The listing builds one solid part. Answer for the finished solid, in the listing's coordinates (mm). Face numbers are marked on the shaded views. Coordinates: 2 decimals unless noted, no trailing zeros. Write each loop counter-clockwise with the first axis right and the second up, starting at its lowest first coordinate (ties: lowest second). Pieces come first, ordered by that corner, then holes. Notation, with made-up numbers: M 53,76.25 L 90,76.25 A12 cw 90,99.25 Z; hole C 32.25,75.25 d3. An arc over 180 degrees is marked long. Answer as CSV lines item,"result".
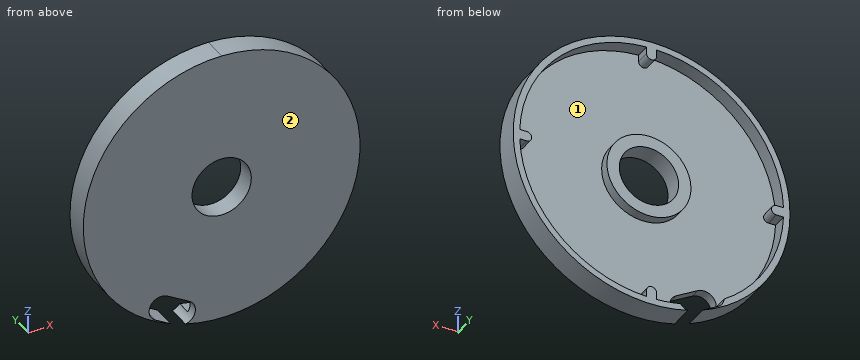
```python
from build123d import *

# Parameters (mm, degrees)
SKETCH_1_R               = 28
EXTRUDE_1_DEPTH          = 2
SKETCH_2_R               = 28
SKETCH_2_R_2             = 26.7
EXTRUDE_3_DEPTH          = 3
EXTRUDE_4_DEPTH          = 3
PATTERN_CIRCULAR_1_COUNT = 4
CUT_EXTRUDE_1_DEPTH      = 5
SKETCH_5_R               = 8.5
SKETCH_5_R_2             = 6
EXTRUDE_5_DEPTH          = 2
SKETCH_6_R               = 6
CUT_EXTRUDE_2_DEPTH      = 2.5


with BuildPart() as part:
    # 草图1 → 凸台-拉伸1 (new body)
    with BuildSketch(Plane(origin=(0, 0, 0), x_dir=(1, 0, 0), z_dir=(0, 1, 0))):
        with Locations(Location((0, 0, 0), (0, 0, 270))):
            Circle(SKETCH_1_R)
    extrude(amount=EXTRUDE_1_DEPTH)

    # 草图2 → 凸台-拉伸3 (add)
    with BuildSketch(Plane(origin=(0, 2, 0), x_dir=(1, 0, 0), z_dir=(0, 1, 0))):
        with Locations(Location((0, 0, 0), (0, 0, 270))):
            Circle(SKETCH_2_R)
        with Locations(Location((0, 0, 0), (0, 0, 270))):
            Circle(SKETCH_2_R_2, mode=Mode.SUBTRACT)
    extrude(amount=EXTRUDE_3_DEPTH)

    # 草图3 → 凸台-拉伸4 (add)
    with BuildSketch(Plane(origin=(0, 2, 0), x_dir=(1, 0, 0), z_dir=(0, 1, 0))):
        with BuildLine():
            Line((1, 26.681266836), (1, 25.262759823))
            ThreePointArc((1, 25.262759823), (0, 24.262759823), (-1, 25.262759823))
            Line((-1, 25.262759823), (-1, 26.681266836))
            ThreePointArc((-1, 26.681266836), (0, 26.7), (1, 26.681266836))
        make_face()
    extrude_4 = extrude(amount=EXTRUDE_4_DEPTH)

    # 阵列(圆周)1: 凸台-拉伸4 ×4 about axis
    pattern_circular_1_axis = Axis((0, 0, 0), (0, 1, 0))
    for i in range(1, PATTERN_CIRCULAR_1_COUNT):
        add(extrude_4.rotate(pattern_circular_1_axis, i * 360 / PATTERN_CIRCULAR_1_COUNT))

    # 草图4 → 切除-拉伸1 (cut, symmetric)
    with BuildSketch(Plane(origin=(0, 2, 0), x_dir=(1, 0, 0), z_dir=(0, 1, 0))):
        with BuildLine():
            Line((-13.418233233, 24.2713603), (-9.042053051, 26.744853446))
            ThreePointArc((-9.042053051, 26.744853446), (-5.635502812, 25.798589491), (-6.581766767, 22.392039253))
            Line((-6.581766767, 22.392039253), (-10.957946949, 19.918546106))
            ThreePointArc((-10.957946949, 19.918546106), (-14.364497188, 20.864810061), (-13.418233233, 24.2713603))
        make_face()
    extrude(amount=CUT_EXTRUDE_1_DEPTH, both=True, mode=Mode.SUBTRACT)

    # 草图5 → 凸台-拉伸5 (add)
    with BuildSketch(Plane(origin=(0, 2, 0), x_dir=(1, 0, 0), z_dir=(0, 1, 0))):
        with Locations(Location((0, 0, 0), (0, 0, 270))):
            Circle(SKETCH_5_R)
        with Locations(Location((0, 0, 0), (0, 0, 270))):
            Circle(SKETCH_5_R_2, mode=Mode.SUBTRACT)
    extrude(amount=EXTRUDE_5_DEPTH)

    # 草图6 → 切除-拉伸2 (cut, symmetric)
    with BuildSketch(Plane(origin=(0, 2, 0), x_dir=(1, 0, 0), z_dir=(0, 1, 0))):
        with Locations(Location((0, 0, 0), (0, 0, 270))):
            Circle(SKETCH_6_R)
    extrude(amount=CUT_EXTRUDE_2_DEPTH, both=True, mode=Mode.SUBTRACT)


solid = part.part
```
Q1. Find section C-C (x = -17). Give the vertices of the cut face in (y, z), and give its area (3 significant figures).
Output:
outline,"M 0,-22.25 L 5,-22.25 L 5,-20.59 L 2,-20.59 L 2,20.59 L 5,20.59 L 5,22.25 L 0,22.25 Z"
area,"99.0 mm2"
Q2. Find section D-D (z = 11). Give the vertices of the cut face in (x, y), and give its area (3 significant figures).
Output:
outline,"M -25.75,0 L 25.75,0 L 25.75,5 L 24.33,5 L 24.33,2 L -24.33,2 L -24.33,5 L -25.75,5 Z"
area,"112 mm2"
Q3. Flat-ended cylindrical pins translate along their axes: pin 1 Ø0.7 at (y, z) = (4, 26) entering from +X; pin 2 Ø18.5 at (x, z) = (2, -4) entering from +Y; pin 3 Ø1.1 at (y, z) = (4, 26) entering from -X; pin 4 Ø11 at (x, z) = (0, 0) entering from -Y. Find the tip coordinate at first contact, or state that the pin passes through.
Output:
pin 1,"x = 11.23"
pin 2,"y = 4"
pin 3,"x = -11.67"
pin 4,"through"
Q4. Find section A-A (y = 2.7). Give the vertices of the cut face in (x, z).
Output:
outline,"M -26.68,-1 L -25.26,-1 A1 ccw -25.26,1 L -26.68,1 A26.7 cw -1,26.68 L -1,25.26 A1 ccw 1,25.26 L 1,26.68 A26.7 cw 26.68,1 L 25.26,1 A1 ccw 25.26,-1 L 26.68,-1 A26.7 cw 1,-26.68 L 1,-25.26 A1 ccw -1,-25.26 L -1,-26.68 A26.7 cw -5.81,-26.06 A2.5 cw -7.33,-27.02 A28 ccw long -10.28,-26.04 L -13.42,-24.27 A2.5 cw -14.68,-22.3 A26.7 cw Z; C 0,0 d17; hole C 0,0 d12"
Q5. Find section B-B (z = 0). Give the vertices of the cut face in (x, y).
Output:
outline,"M -28,0 L -6,0 L -6,4 L -8.5,4 L -8.5,2 L -24.26,2 L -24.26,5 L -28,5 Z; M 6,0 L 28,0 L 28,5 L 24.26,5 L 24.26,2 L 8.5,2 L 8.5,4 L 6,4 Z"
Q6. The mould has two halves that part along Z. Classify the marked faces 1 and 2: pulls with the +Z half, pulls with the -Z half, needs draft (parallel to the pull), parting line crosses it, or undercut.
Output:
face 1,"undercut"
face 2,"needs draft"
Q7. Straight lines are drawn through the part: line 1 (X direction, y = 2.75, z = 0); line 2 (X direction, y = 1.4, z = 0); line 3 (Z direction, x = 7.5, y = 2.05). For each, find the intervals that lie inside material, in ascending order.
Output:
line 1,"-28 to -24.26, -8.5 to -6, 6 to 8.5, 24.26 to 28"
line 2,"-28 to -6, 6 to 28"
line 3,"-26.98 to -25.62, -4 to 4, 25.62 to 26.98"
